Source: CAD feature listing. Evaluate the final solid. Frame: model axes, mm. A direction names the side the tool comes from. Round coordinates to 2 decimals unless told otherwise and drop trailing zeros. Answer in a Markdown table with one row per item.
from build123d import *

# Parameters (mm, degrees)
F2_R     = 8
F3_DEPTH = 12.701
F4_R     = 8


with BuildPart() as f1:
    # F0 (on Right) → F1 (revolve)
    with BuildSketch(Plane.YZ):
        with BuildLine():
            Line((-12.7, 15), (-12.7, 0))
            Line((-12.7, 0), (-3.35, 0))
            Line((-3.35, 0), (-3.35, 15))
            add(Edge.make_bspline(
                [(-3.35, 15), (-3.35, 20.828191), (0, 22.027135), (0, 27.5)],
                knots=[0, 0, 0, 0, 12.941117, 12.941117, 12.941117, 12.941117], degree=3))
            Line((0, 27.5), (0, 35.5))
            Line((0, 35.5), (-6.35, 35.5))
            Line((-6.35, 35.5), (-6.35, 27.5))
            ThreePointArc((-6.35, 27.5), (-11.021488, 22.010216), (-12.7, 15))
        make_face()
    revolve(axis=Axis((0, -9.5, 0), (0, -1, 0)))

    # F2 (on face) → F3 (cut, through all)
    with BuildSketch(Plane.XZ.offset(12.7)):
        Circle(F2_R)
    extrude(amount=-F3_DEPTH, mode=Mode.SUBTRACT)

    # F4
    f4_edges = [f1.edges().sort_by_distance(p)[0] for p in [
        (0, -6.35, -27.5),
    ]]
    fillet(f4_edges, radius=F4_R)


solid = f1.part
Q1. Contact query for flat-ended pins moving along their axis: pin 1 Ø4 at (x, y) = (8.5, -9) entering from -Z; pin 2 Ø2 at (x, y) = (-25, -2) entering from +Z; pin 3 Ø3 at (y, z) = (-6, 23.5) entering from +X. Output: stop coordinate, or through.
Solutions:
| item | result |
|---|---|
| pin 1 | stops at z = -26.61 |
| pin 2 | stops at z = 26.16 |
| pin 3 | stops at x = 27.86 |
Q2. Pull-direction query (Z, two-part tool) for faces 1 (the cylindrical face through (34.656, -3.219, -7.696)), 2 (the flat face through (6, -3.35, -6)), 3 (the flat face through (21, 0, -18)); classes: pulls with the +Z half, pulls with the -Z half, needs draft (parallel to the pull), parting line crosses it, or undercut.
Solutions:
| item | result |
|---|---|
| face 1 | parting line crosses it |
| face 2 | undercut |
| face 3 | needs draft |
Q3. Access query for faces 4 (the cylindrical face through (-1.73, -8.09, -7.81)), 5 (the flat face through (31.4, -6.35, -0.2)). Directions: +Z, -Z, +X, -X, +Y, -Y. A direction counts if a zero-diameter tool reaches every point of the face in a straight line with its end or side. Return the directions, or none.
Solutions:
| item | result |
|---|---|
| face 4 | +Y, -Y |
| face 5 | -Y |
Q4. Material intervals for probe 1 along Z at (x, y) = (0, -5.25); probe 2 along Y at (x, z) = (-10.5, 9.5); probe 3 along X at (y, z) = (-5, -5.5), sorted ascending.
Solutions:
| item | result |
|---|---|
| probe 1 | z = -35.5 to -8, 8 to 35.5 |
| probe 2 | y = -12.7 to -3.35 |
| probe 3 | x = -35.07 to -5.81, 5.81 to 35.07 |
